Input: part model. Units: mm. Frame: model coordinates. A direction names the side the tool comes from. Round coordinates to 2 decimals unless told otherwise and drop trailing zeros. Loops run counter-clockwise (first coordinate to the right, second up) from the corner with the lowest first, then second, coordinate; pieces in that order, holes last. Notation, with made-up numbers: M 81.5,38 L 101.5,38 A19 ccw 101.5,65 Z; hole C 32,-18 d7. An arc over 180 degrees is marked long. Return JSON: item names as keys, results as strings. Group by question number.
1) Section B-B (y = 27.5). Output: boundary loops of the cut face in (x, z).
2) Section A-A (z = 3). Output: boundary loops of the cut face in (x, y), plus the area to 3 significant figures.
3) Section D-D (z = -11). Output: boundary loops of the cut face in (x, y), plus the area to 3 significant figures.
4) Material intervals for line 1 (Z direction, x = -6, y = 27); line 2 (X direction, y = 19, z = 7); line 3 (Z direction, x = 6.5, y = 11), sorted ascending. Write a range as from..to.
5) Section C-C (x = 43.5). Output: boundary loops of the cut face in (y, z).
6) Mould query, pull axis Z, two halves, no side actions, for faces 1 (the face through (32, 10, -36)), 2 (the face through (-5, 23, 25.654)), 3 (the face through (88.675, -35.541, -15.914)). Classes: +Z half, -Z half, draft (parallel to the pull), parting line (faces both ways), or undercut.
7) Access query for faces 4 (the face through (44, 19.244, -24)), 5 (the face through (74.49, -4.28, -23.57)), 6 (the face through (53, 12, -19.346)), 7 (the face through (79, -12, -4.346)). Directions: +Z, -Z, +X, -X, +Y, -Y. A direction counts if a zero-diameter tool reaches every point of the face in a straight line with its end or side. Return the directions, or none.
8) Contact query for flat-ended pins moving along their axis: P1, Ø12.5, axis at x = 73, y = -7.5, coming from the +Z side; P2, Ø6, axis at y = -28.5, z = -37, coming from the -X side; P3, Ø3, axis at y = 15.5, z = -32, coming from the +X side. Output: stop coordinate, or through.
from build123d import *

# Parameters (mm, degrees)
SKETCH1_W           = 69
SKETCH1_H           = 45
BOSS_EXTRUDE1_DEPTH = 10
BOSS_EXTRUDE2_DEPTH = 69
CUT_EXTRUDE1_DEPTH  = 69
SKETCH5_W           = 10
SKETCH5_H           = 40.367791419
CUT_EXTRUDE2_DEPTH  = 30
SKETCH6_R           = 19.5
BOSS_EXTRUDE3_DEPTH = 12
CUT_EXTRUDE3_START  = -12
CUT_EXTRUDE3_DEPTH  = 12
BOSS_EXTRUDE4_START = 3
SKETCH8_R           = 19.5
BOSS_EXTRUDE4_DEPTH = 3
CUT_EXTRUDE4_REACH  = 124.458
SKETCH9_R           = 8
BOSS_EXTRUDE5_START = -5
BOSS_EXTRUDE5_DEPTH = 10
CUT_EXTRUDE5_REACH  = 132.828
SKETCH14_R          = 8


# Read off the part's stored shape, not the designer's step: Boss-Extrude5
with BuildPart() as part:
    # Sketch1 → Boss-Extrude1 (new body)
    with BuildSketch(Plane(origin=(0, 0, 0), x_dir=(0, 0, -1), z_dir=(1, 0, 0))):
        with Locations((8.845653905, 22.5)):
            Rectangle(SKETCH1_W, SKETCH1_H)
    extrude(amount=-BOSS_EXTRUDE1_DEPTH)

    # Sketch2 → Boss-Extrude2 (add)
    with BuildSketch(Plane.XY.offset(25.654346095)):
        with BuildLine():
            Line((64, 10), (0, 10))
            Line((0, 10), (0, 0))
            Line((0, 0), (44.854374374, 0))
            Line((44.854374374, 0), (64, 0))
            ThreePointArc((64, 0), (74.606601718, -4.393398282), (79, -15))
            Line((79, -15), (79, -55.367791419))
            Line((79, -55.367791419), (89, -55.367791419))
            Line((89, -55.367791419), (89, -15))
            ThreePointArc((89, -15), (81.67766953, 2.67766953), (64, 10))
        make_face()
    extrude(amount=-BOSS_EXTRUDE2_DEPTH)

    # Sketch4 → Cut-Extrude1 (cut)
    with BuildSketch(Plane(origin=(0, 10, 0), x_dir=(1, 0, 0), z_dir=(0, 1, 0))):
        with BuildLine():
            ThreePointArc((30.643579789, 4.338749862), (9.015569982, -4.21481026), (0, -25.654346095))
            Line((0, -25.654346095), (64, -25.654346095))
            Line((64, -25.654346095), (64, 4.338749862))
            Line((64, 4.338749862), (30.643579789, 4.338749862))
        make_face()
    extrude(amount=-CUT_EXTRUDE1_DEPTH, mode=Mode.SUBTRACT)

    # Sketch5 → Cut-Extrude2 (cut)
    with BuildSketch(Plane.XY.offset(25.654346095)):
        with BuildLine():
            Line((89, -15), (79, -15))
            ThreePointArc((79, -15), (74.606601718, -4.393398282), (64, 0))
            Line((64, 0), (64, 10))
            ThreePointArc((64, 10), (81.67766953, 2.67766953), (89, -15))
        make_face()
        with Locations((84, -35.18389571)):
            Rectangle(SKETCH5_W, SKETCH5_H)
    extrude(amount=-CUT_EXTRUDE2_DEPTH, mode=Mode.SUBTRACT)

    # Sketch6 → Boss-Extrude3 (add)
    with BuildSketch(Plane(origin=(89, 0, 0), x_dir=(0, 0, -1), z_dir=(1, 0, 0))):
        with Locations(Location((23.845653905, -34.5, 0), (0, 0, 90))):
            Circle(SKETCH6_R)
    extrude(amount=BOSS_EXTRUDE3_DEPTH)

    # Sketch7 → Cut-Extrude3 (cut)
    with BuildSketch(Plane(origin=(89, 0, 0), x_dir=(0, 0, -1), z_dir=(1, 0, 0)).offset(CUT_EXTRUDE3_START)):
        with BuildLine():
            Line((4.345653905, -34.5), (4.345653905, -55.367791419))
            Line((4.345653905, -55.367791419), (43.345653905, -55.367791419))
            Line((43.345653905, -55.367791419), (43.345653905, -34.5))
            ThreePointArc((43.345653905, -34.5), (23.845653905, -54), (4.345653905, -34.5))
        make_face()
    extrude(amount=CUT_EXTRUDE3_DEPTH, mode=Mode.SUBTRACT)

    # Sketch8 → Boss-Extrude4 (add)
    with BuildSketch(Plane.ZY.offset(-79).offset(BOSS_EXTRUDE4_START)):
        with Locations((-23.845653905, -34.5)):
            Circle(SKETCH8_R)
    extrude(amount=-BOSS_EXTRUDE4_DEPTH)

    # Sketch9 → Cut-Extrude4 (cut, up to next)
    with BuildSketch(Plane(origin=(0, 0, 0), x_dir=(0, 0, -1), z_dir=(1, 0, 0)), mode=Mode.PRIVATE) as cut_extrude4_sk1:
        with Locations((-3.654346095, 27.5)):
            Circle(SKETCH9_R)
    cut_extrude4_tool1 = extrude(cut_extrude4_sk1.sketch, amount=-CUT_EXTRUDE4_REACH, mode=Mode.PRIVATE) & part.part
    add(cut_extrude4_tool1.solids().sort_by_distance((0, 27.5, 3.654346))[0], mode=Mode.SUBTRACT)

    # Boss-Extrude5 outline → Boss-Extrude5 (add)
    with BuildSketch(Plane(origin=(0, 0, -24.345653905), x_dir=(-1, 0, 0), z_dir=(0, 0, -1)).offset(BOSS_EXTRUDE5_START)):
        with BuildLine():
            Line((0, 10), (0, 43.487506986))
            ThreePointArc((0, 43.487506986), (-7.58031637, 26.300702433), (-24.988559207, 19.243753493))
            Line((-24.988559207, 19.243753493), (-64, 19.243753493))
            ThreePointArc((-64, 19.243753493), (-88.701898796, 9.482823843), (-99, -15))
            Line((-99, -15), (-99, -34.5))
            Line((-99, -34.5), (-89, -34.5))
            Line((-89, -34.5), (-89, -15))
            ThreePointArc((-89, -15), (-81.67766953, 2.67766953), (-64, 10))
            Line((-64, 10), (0, 10))
        make_face()
    extrude(amount=BOSS_EXTRUDE5_DEPTH)

    # Sketch14 → Cut-Extrude5 (cut, up to next)
    with BuildSketch(Plane(origin=(101, 0, 0), x_dir=(0, 0, -1), z_dir=(1, 0, 0)), mode=Mode.PRIVATE) as cut_extrude5_sk1:
        with Locations(Location((23.845653905, -34.5, 0), (0, 0, 90))):
            Circle(SKETCH14_R)
    cut_extrude5_tool1 = extrude(cut_extrude5_sk1.sketch, amount=-CUT_EXTRUDE5_REACH, mode=Mode.PRIVATE) & part.part
    add(cut_extrude5_tool1.solids().sort_by_distance((101, -34.5, -23.845654))[0], mode=Mode.SUBTRACT)


solid = part.part
Returned:
{
 "1": {"outline": "M -10,-43.35 L 0,-43.35 L 0,-29.35 L 6.42,-29.35 L 6.42,-19.35 L 0,-19.35 L 0,-4.35 L -10,-4.35 Z; M -10,11.65 L 0,11.65 L 0,25.65 L -10,25.65 Z"},
 "2": {"outline": "M -10,0 L 10.33,0 L 10.33,10 L 0,10 L 0,19.53 L -10,19.53 Z; M -10,35.47 L 0,35.47 L 0,45 L -10,45 Z", "area": "394 mm^2"},
 "3": {"outline": "M -10,0 L 64,0 A15 cw 79,-15 L 79,-19.83 L 76,-19.83 L 76,-49.17 L 101,-49.17 L 101,-19.83 L 89,-19.83 L 89,-15 A25 ccw 64,10 L 0,10 L 0,45 L -10,45 Z", "area": "2,190 mm^2"},
 "4": {"line 1": "z = -43.35..-4.33, 11.64..25.65", "line 2": "x = -10..0", "line 3": "z = -29.35..-19.35"},
 "5": {"outline": "M 0,-43.35 L 10,-43.35 L 10,-29.35 L 19.24,-29.35 L 19.24,-19.35 L 10,-19.35 L 10,-4.34 L 0,-4.34 Z"},
 "6": {"face 1": "draft", "face 2": "+Z half", "face 3": "undercut"},
 "7": {"face 4": "+Z, -Z, +X, +Y", "face 5": "+Z, -Z, -X", "face 6": "+Z, +X, +Y", "face 7": "+Z, +X, +Y, -Y"},
 "8": {"P1": "stops at z = -4.35", "P2": "stops at x = 76", "P3": "stops at x = 0"}
}
